```python
from build123d import *

# Parameters (mm, degrees)
F0_R     = 1.5
F1_DEPTH = 60
F2_DEPTH = 2.7


with BuildPart() as f1:
    # F0 (on Front) → F1 (new body)
    with BuildSketch(Plane.XZ):
        Circle(F0_R)
    extrude(amount=F1_DEPTH)

    # F0 (on Front) → F2 (join)
    with BuildSketch(Plane.XZ):
        Polygon((-0.82392, 2.64597), (-2.703437, 0.609449), (-1.879517, -2.03652), (0.82392, -2.64597), (2.703437, -0.609449), (1.879517, 2.03652), align=None)
        Circle(F0_R, mode=Mode.SUBTRACT)
        Circle(F0_R)
    extrude(amount=-F2_DEPTH)


solid = f1.part
```
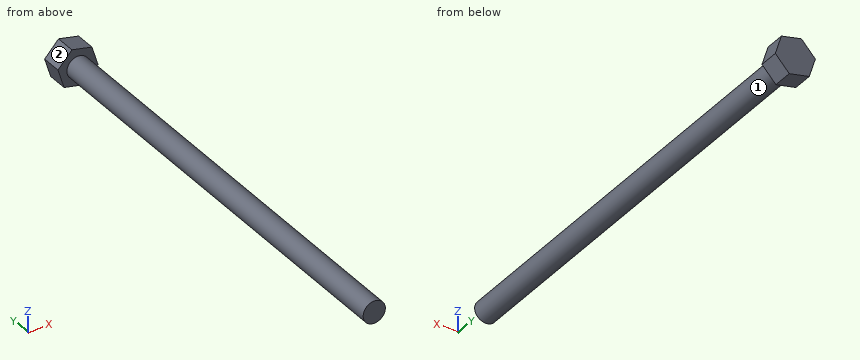
Check sheet for the modelled part. Datum: model origin and axes. Units: mm. Face numbers are marked on the shaded views. A direction names the side the tool comes from. Round coordinates to 2 decimals unless told otherwise and drop trailing zeros. Loops run counter-clockwise (first coordinate to the right, second up) from the corner with the lowest first, then second, coordinate; pieces in that order, holes last. Notation, with made-up numbers: (43, 22) - (58, 22) arc R12 cw to (58, 44) - close; hole circle Ø5 at (-1.5, 34.25). An arc over 180 degrees is marked (long way). Write item = value, one per line. Start each with the question number.
Q1. Section check C-C (y = -52). Record the boundary of the cut face in (x, z), plus the area to 3 significant figures.
Q2. Section check A-A (z = 0). Record the boundary of the cut face in (x, y).
Q3. Access from +Z, -Z, +X, -X, +Y, -Y to the whole of each face (thin tool, end or side, straight path). Record for the marked faces 1 and 2.
Q4. Section check B-B (x = 0). Record the boundary of the cut face in (y, z).
Q5. Depth check by flat-ended pin: P1, Ø1.5, axis at x = 1.5, y = -27.5, coming from the +Z side; P2, Ø1.5, axis at x = 0, y = -5.5, coming from the -Z side; P3, Ø2, axis at y = -19, z = 1.5, coming from the -X side. Enter the tip coordinate at first touch or a pass-through.
Q6. Thickness scan on L1, parallel to Y at x = -1.85, z = -0.6; L2, parallel to Z at x = 0, y = -55; L3, parallel to X at y = -24, z = -0.15. Record the ranges inside material, lowest first.
Derived:
q1.outline = circle Ø3 at (0, 0)
q1.area = 7.07 mm^2
q2.outline = (-2.51, 0) - (-1.5, 0) - (-1.5, -60) - (1.5, -60) - (1.5, 0) - (2.51, 0) - (2.51, 2.7) - (-2.51, 2.7) - close
q3.face_1 = -Y
q3.face_2 = +Z, -X, +Y, -Y
q4.outline = (-60, -1.5) - (0, -1.5) - (0, -2.46) - (2.7, -2.46) - (2.7, 2.46) - (0, 2.46) - (0, 1.5) - (-60, 1.5) - close
q5.P1 = 1.3
q5.P2 = -1.5
q5.P3 = -1.41
q6.L1 = 0 to 2.7
q6.L2 = -1.5 to 1.5
q6.L3 = -1.49 to 1.49
